Autodesk Fusion 360 part; units mm, degrees
sketch "panel" plane through (0, 0, 0) normal (0, 0, 1) x (1, 0, 0)
  line L0 (62.8541, 263.5001) -> (357.1459, 263.5001)
  line L1 (357.1459, 263.5001) -> (357.1459, 33.5001)
  line L2 (357.1459, 33.5001) -> (62.8541, 33.5001)
  line L3 (62.8541, 33.5001) -> (62.8541, 263.5001)
  line L4 (137.8887, 199.6854) -> (139.7122, 197.8619)
  line L5 (139.7122, 199.6854) -> (137.8887, 197.8619)
  line L6 (167.3878, 199.4554) -> (169.2113, 197.6319)
  line L7 (169.2113, 199.4554) -> (167.3878, 197.6319)
  line L8 (193.5289, 185.7844) -> (195.3524, 183.9609)
  line L9 (195.3524, 185.7844) -> (193.5289, 183.9609)
  line L10 (220.9942, 199.2964) -> (222.8177, 197.4729)
  line L11 (222.8177, 199.2964) -> (220.9942, 197.4729)
  line L12 (247.5472, 212.1984) -> (249.3707, 210.3749)
  line L13 (249.3707, 212.1984) -> (247.5472, 210.3749)
  line L14 (277.0202, 210.8714) -> (278.8437, 209.0479)
  line L15 (278.8437, 210.8714) -> (277.0202, 209.0479)
  line L16 (306.1132, 205.9884) -> (307.9366, 204.1649)
  line L17 (307.9366, 205.9884) -> (306.1132, 204.1649)
  line L18 (304.0832, 175.4464) -> (305.9067, 173.6229)
  line L19 (305.9067, 175.4464) -> (304.0832, 173.6229)
  line L20 (274.9902, 180.3294) -> (276.8136, 178.5059)
  line L21 (276.8136, 180.3294) -> (274.9902, 178.5059)
  line L22 (245.5172, 181.6564) -> (247.3407, 179.8329)
  line L23 (247.3407, 181.6564) -> (245.5172, 179.8329)
  line L24 (218.9642, 168.7544) -> (220.7877, 166.9309)
  line L25 (220.7877, 168.7544) -> (218.9642, 166.9309)
  line L26 (230.8722, 141.9414) -> (232.6957, 140.1179)
  line L27 (232.6957, 141.9414) -> (230.8722, 140.1179)
  line L28 (173.1491, 148.1874) -> (174.9726, 146.3639)
  line L29 (174.9726, 148.1874) -> (173.1491, 146.3639)
  line L30 (200.3572, 129.9534) -> (202.1807, 128.1299)
  line L31 (202.1807, 129.9534) -> (200.3572, 128.1299)
  line L32 (108.0433, 242.9744) -> (109.8668, 241.1509)
  line L33 (109.8668, 242.9744) -> (108.0433, 241.1509)
  line L34 (130.0434, 242.9744) -> (131.8669, 241.1509)
  line L35 (131.8668, 242.9744) -> (130.0434, 241.1509)
  line L36 (152.0434, 242.9744) -> (153.8668, 241.1509)
  line L37 (153.8668, 242.9744) -> (152.0434, 241.1509)
  line L38 (174.0434, 242.9744) -> (175.8668, 241.1509)
  line L39 (175.8668, 242.9744) -> (174.0434, 241.1509)
  line L40 (75.8193, 250.5344) -> (77.6428, 248.7109)
  line L41 (77.6428, 250.5344) -> (75.8193, 248.7109)
  line L42 (75.8428, 149.3114) -> (77.6663, 147.4879)
  line L43 (77.6663, 149.3114) -> (75.8428, 147.4879)
  line L44 (75.8428, 48.1124) -> (77.6663, 46.2889)
  line L45 (77.6663, 48.1124) -> (75.8428, 46.2889)
  line L46 (209.1882, 250.5114) -> (211.0117, 248.6879)
  line L47 (211.0117, 250.5114) -> (209.1882, 248.6879)
  line L48 (342.5342, 149.3114) -> (344.3576, 147.4879)
  line L49 (344.3576, 149.3114) -> (342.5342, 147.4879)
  line L50 (342.5342, 250.5114) -> (344.3576, 248.6879)
  line L51 (344.3576, 250.5114) -> (342.5342, 248.6879)
  line L52 (342.5342, 48.1124) -> (344.3576, 46.2889)
  line L53 (344.3576, 48.1124) -> (342.5342, 46.2889)
  line L54 (209.1882, 48.1124) -> (211.0117, 46.2889)
  line L55 (211.0117, 48.1124) -> (209.1882, 46.2889)
  circle A0 centre (76.731, 249.6226) radius 2.3
  circle A1 centre (76.7545, 148.3996) radius 2.3
  circle A2 centre (76.7545, 47.2006) radius 2.3
  circle A3 centre (210.0999, 249.5996) radius 2.3
  circle A4 centre (343.4459, 249.5996) radius 2.3
  circle A5 centre (343.4459, 148.3996) radius 2.3
  circle A6 centre (343.4459, 47.2006) radius 2.3
  circle A7 centre (210.0999, 47.2006) radius 2.3
  circle A8 centre (138.8004, 198.7736) radius 12.3
  circle A9 centre (168.2995, 198.5436) radius 12.3
  circle A10 centre (194.4406, 184.8726) radius 12.3
  circle A11 centre (219.8759, 167.8426) radius 12.3
  circle A12 centre (221.9059, 198.3846) radius 12.3
  circle A13 centre (248.4589, 211.2866) radius 12.3
  circle A14 centre (246.4289, 180.7446) radius 12.3
  circle A15 centre (275.9019, 179.4176) radius 12.3
  circle A16 centre (277.9319, 209.9596) radius 12.3
  circle A17 centre (307.0249, 205.0766) radius 12.3
  circle A18 centre (304.9949, 174.5346) radius 12.3
  circle A19 centre (174.0608, 147.2756) radius 12.3
  circle A20 centre (231.7839, 141.0296) radius 12.3
  circle A21 centre (201.2689, 129.0416) radius 15.3
  circle A22 centre (108.9551, 242.0626) radius 8.3
  circle A23 centre (130.9551, 242.0626) radius 8.3
  circle A24 centre (152.9551, 242.0626) radius 8.3
  circle A25 centre (174.9551, 242.0626) radius 8.3
  line L56 (222.9609, 104.4851) -> (310.7209, 104.4851) construction
  line L57 (310.7209, 104.4851) -> (310.7209, 67.5251) construction
  line L58 (310.7209, 67.5251) -> (222.9609, 67.5251) construction
  line L59 (222.9609, 67.5251) -> (222.9609, 104.4851) construction
  line L60 (218.5359, 108.5101) -> (315.1459, 108.5101) construction
  line L61 (315.1459, 108.5101) -> (315.1459, 63.5001) construction
  line L62 (315.1459, 63.5001) -> (218.5359, 63.5001) construction
  line L63 (218.5359, 63.5001) -> (218.5359, 108.5101) construction
  line L64 (222.9609, 104.4851) -> (310.7209, 67.5251) construction
  line L65 (310.7209, 104.4851) -> (222.9609, 67.5251) construction
  line L66 (266.8409, 67.5251) -> (266.8409, 104.4851) construction
  line L67 (310.7209, 86.0051) -> (222.9609, 86.0051) construction
  line L68 (357.1459, 33.5001) -> (315.1459, 33.5001) construction
  line L69 (315.1459, 33.5001) -> (315.1459, 63.5001) construction
  line L70 (315.1459, 63.5001) -> (357.1459, 63.5001) construction
  line L71 (357.1459, 63.5001) -> (357.1459, 33.5001) construction
  circle A26 centre (222.9609, 104.4851) radius 1.6 construction
  circle A27 centre (222.9609, 67.5251) radius 1.6 construction
  circle A28 centre (310.7209, 67.5251) radius 1.6 construction
  circle A29 centre (310.7209, 104.4851) radius 1.6 construction
  circle A30 centre (222.9609, 104.4851) radius 4.025
  circle A31 centre (222.9609, 67.5251) radius 4.025
  circle A32 centre (310.7209, 67.5251) radius 4.025
  circle A33 centre (310.7209, 104.4851) radius 4.025
  line L72 (210.0999, 47.2006) -> (220.0999, 47.2006) construction
  line L73 (220.0999, 47.2006) -> (220.0999, 57.2006) construction
  line L74 (220.0999, 57.2006) -> (210.0999, 57.2006) construction
  line L75 (210.0999, 57.2006) -> (210.0999, 47.2006) construction
  line L76 (343.4459, 47.2006) -> (333.4459, 47.2006) construction
  line L77 (333.4459, 47.2006) -> (333.4459, 57.2006) construction
  line L78 (333.4459, 57.2006) -> (343.4459, 57.2006) construction
  line L79 (343.4459, 57.2006) -> (343.4459, 47.2006) construction
  line L80 (214.2369, 112.8091) -> (319.4449, 112.8091)
  line L81 (319.4449, 112.8091) -> (319.4449, 59.2006)
  line L82 (319.4449, 59.2006) -> (214.2369, 59.2006)
  line L83 (214.2369, 59.2006) -> (214.2369, 112.8091)
  dimension "d1" = 4.6
  dimension "d2" = 4.6
  dimension "d3" = 4.6
  dimension "d4" = 4.6
  dimension "d5" = 4.6
  dimension "d6" = 4.6
  dimension "d7" = 4.6
  dimension "d8" = 4.6
  dimension "d9" = 24.6
  dimension "d10" = 24.6
  dimension "d11" = 24.6
  dimension "d12" = 24.6
  dimension "d13" = 24.6
  dimension "d14" = 24.6
  dimension "d15" = 24.6
  dimension "d16" = 24.6
  dimension "d17" = 24.6
  dimension "d18" = 24.6
  dimension "d19" = 24.6
  dimension "d20" = 24.6
  dimension "d21" = 24.6
  dimension "d22" = 30.6
  dimension "d23" = 16.6
  dimension "d24" = 16.6
  dimension "d25" = 16.6
  dimension "d26" = 16.6
  dimension "d31" = 36.96
  dimension "d32" = 87.76
  dimension "d33" = 96.61
  dimension "d34" = 45.01
  dimension "d35" = 42
  dimension "d36" = 30
  dimension "d37" = 3.2
  dimension "d38" = 3.2
  dimension "d39" = 3.2
  dimension "d40" = 3.2
  dimension "d41" = 10
  dimension "d42" = 10
  dimension "d43" = 10
  dimension "d44" = 10
  dimension "d45" = 2
  dimension "d47" = 4.299
  dimension "d48" = 4.299
  dimension "d73" = 4.299
extrude "Extrude1" add sketch "panel" along normal blind 1.5 contours L0 L1 L2 L3 | A30 | A31 | A32 | A33 | L80 L81 L82 L83
fillet "Fillet1" radius 2 4 edges at (62.8541, 33.5001, 0.75) (62.8541, 263.5001, 0.75) (357.1459, 33.5001, 0.75) (357.1459, 263.5001, 0.75)
extrude "Extrude2" cut sketch "panel" along normal blind 0.5 contours L80 L81 L82 L83
extrude "Extrude3" add 4 faces at (311.7044, 105.7976, 0) (223.2594, 103.1771, 0) (223.2594, 66.2171, 0) (311.9888, 66.3632, 0) along direction (0, 0, -1) blind 1.5
hole "Hole1" at (310.7209, 104.4851, -1.5) direction (0, 0, 1) diameter 2.529 depth 1.5 tip angle 118
hole "Hole2" at (310.7209, 67.5251, -1.5) direction (0, 0, 1) diameter 2.529 depth 1.5 tip angle 118
hole "Hole3" at (222.9609, 104.4851, -1.5) direction (0, 0, 1) diameter 2.529 depth 1.5 tip angle 118
hole "Hole4" at (222.9609, 67.5251, -1.5) direction (0, 0, 1) diameter 2.529 depth 1.5 tip angle 118
fillet "Fillet2" radius 2 4 edges at (319.4449, 112.8091, 0.25) (214.2369, 112.8091, 0.25) (214.2369, 59.2006, 0.25) (319.4449, 59.2006, 0.25)
Check sheet for the modelled part. Datum: model origin and axes. Units: mm. A direction names the side the tool comes from. Coordinates: 2 decimals unless noted, no trailing zeros. Loops run counter-clockwise (first coordinate to the right, second up) from the corner with the lowest first, then second, coordinate; pieces in that order, holes last. Notation, with made-up numbers: (23, 0.25) -> (44, 0.25) arc R18 ccw to (44, 10.25) -> close; hole circle Ø11 at (36.25, 88.25). An arc over 180 degrees is marked (long way). Answer in a Markdown table with one row per item.
1. Sectioned sample at C-C, the plane y = 88. Record the boundary of the cut face in (x, z), then the cut area to 3 significant figures.
Check values:
| item | result |
|---|---|
| outline | (62.85, 0) -> (214.24, 0) -> (214.24, 0.5) -> (319.44, 0.5) -> (319.44, 0) -> (357.15, 0) -> (357.15, 1.5) -> (62.85, 1.5) -> close |
| area | 389 mm2 |
2. Sectioned sample at D-D, the plane x = 334. Record the boundary of the cut face in (y, z), then the cut area to 3 significant figures.
Check values:
| item | result |
|---|---|
| outline | (33.5, 0) -> (263.5, 0) -> (263.5, 1.5) -> (33.5, 1.5) -> close |
| area | 345 mm2 |
3. Material ranges on line 1 along X through (y, z) = (241.5, 0.8); line 2 along X through (y, z) = (157, 0.35); line 3 along X through (y, z) = (158.5, 0.7), recorded low to high. Write a range as [from, to].
Check values:
| item | result |
|---|---|
| line 1 | x = [62.85, 100.67], [117.24, 122.67], [139.24, 144.67], [161.24, 166.67], [183.24, 357.15] |
| line 2 | x = [62.85, 166.53], [181.59, 214.07], [225.68, 357.15] |
| line 3 | x = [62.85, 169.03], [179.09, 211.88], [227.88, 357.15] |
4. Sectioned sample at B-B, the plane x = 239.5. Record the boundary of the cut face in (y, z).
Check values:
| item | result |
|---|---|
| outline | (33.5, 0) -> (59.2, 0) -> (59.2, 0.5) -> (112.81, 0.5) -> (112.81, 0) -> (131.45, 0) -> (131.45, 1.5) -> (33.5, 1.5) -> close; (150.61, 0) -> (170.58, 0) -> (170.58, 1.5) -> (150.61, 1.5) -> close; (190.91, 0) -> (202.86, 0) -> (202.86, 1.5) -> (190.91, 1.5) -> close; (219.71, 0) -> (263.5, 0) -> (263.5, 1.5) -> (219.71, 1.5) -> close |
5. Release check for a two-part mould opening along Y. For faces 3 (the face through (208, 150, 1.5)), 4 (the face through (306.7, 67.35, -0.51)), 5 (the face through (165, 138.96, 0.74)) record: released by +Y, released by -Y, zero draft, split by the parting line, or undercut.
Check values:
| item | result |
|---|---|
| face 3 | zero draft |
| face 4 | undercut |
| face 5 | undercut |
6. Sectioned sample at A-A, the plane z = -0.85. Give the number of separate pieces and of enclosed holes in the cut face, then the cut area to 3 significant figures.
Check values:
| item | result |
|---|---|
| separate pieces | 4 |
| enclosed holes | 4 |
| area | 183 mm2 |
7. Access from +Z, -Z, +X, -X, +Y, -Y to the whole of each face (thin tool, end or side, straight path). Record for faces 1 (the face through (266, 86, 0.5)), 2 (the face through (225, 68, -1.5)).
Check values:
| item | result |
|---|---|
| face 1 | -Z |
| face 2 | -Z, +X, -X, +Y, -Y |
